```python
from build123d import *

# Parameters (mm, degrees)
SKETCH1_R           = 1.5
BOSS_EXTRUDE1_DEPTH = 3
BOSS_EXTRUDE2_START = 22.5
SKETCH2_W           = 3.5
SKETCH2_H           = 6
BOSS_EXTRUDE2_DEPTH = 29
SKETCH4_R           = 1.5
BOSS_EXTRUDE5_DEPTH = 1
CHAMFER2_SIZE       = 2
CHAMFER2_SIZE2      = 3.464101615
SKETCH3_W           = 24
SKETCH3_H           = 29
SKETCH3_R           = 11
BOSS_EXTRUDE4_DEPTH = 7
CHAMFER3_SIZE       = 2
SKETCH5_R           = 2
BOSS_EXTRUDE6_DEPTH = 14
CHAMFER5_SIZE       = 5


# Read off the part's stored shape, not the designer's step: Mirror1
with BuildPart() as part:
    # Sketch1 → Boss-Extrude1 (new body)
    with BuildSketch(Plane(origin=(0, 0, 0), x_dir=(1, 0, 0), z_dir=(0, 1, 0))):
        Polygon((-6, 17), (-3, 20), (3, 20), (6, 17), (6, -17), (3, -20), (-3, -20), (-6, -17), align=None)
        with Locations(Location((0, 14, 0), (0, 0, 270))):
            Circle(SKETCH1_R, mode=Mode.SUBTRACT)
        with Locations(Location((0, -14, 0), (0, 0, 270))):
            Circle(SKETCH1_R, mode=Mode.SUBTRACT)
    extrude(amount=BOSS_EXTRUDE1_DEPTH)

    # Sketch2 → Boss-Extrude2 (add)
    with BuildSketch(Plane(origin=(0, 3, 0), x_dir=(1, 0, 0), z_dir=(0, 1, 0)).offset(BOSS_EXTRUDE2_START)):
        with Locations((-7.75, 9)):
            Rectangle(SKETCH2_W, SKETCH2_H)
        with Locations((-7.75, -9)):
            Rectangle(SKETCH2_W, SKETCH2_H)
    extrude(amount=-BOSS_EXTRUDE2_DEPTH)

    # Sketch4 → Boss-Extrude5 (add)
    with BuildSketch(Plane(origin=(0, 3, 0), x_dir=(1, 0, 0), z_dir=(0, 1, 0))):
        Polygon((-3, 20), (-6, 17), (-6, 12), (-6, 6), (-6, -6), (-6, -12), (-6, -17), (-3, -20), (3, -20), (6, -17), (6, 17), (3, 20), align=None)
        with Locations(Location((0, 14, 0), (0, 0, 270))):
            Circle(SKETCH4_R, mode=Mode.SUBTRACT)
        with Locations(Location((0, -14, 0), (0, 0, 270))):
            Circle(SKETCH4_R, mode=Mode.SUBTRACT)
    extrude(amount=BOSS_EXTRUDE5_DEPTH)

    # Chamfer2
    chamfer2_edges = [part.edges().sort_by_distance(p)[0] for p in [
        (-6, 0, -9),
        (-6, 0, 9),
    ]]
    chamfer2_side = [part.faces().sort_by_distance(p)[0] for p in [
        (0, 0, 0),
    ]]
    chamfer(chamfer2_edges, length=CHAMFER2_SIZE, length2=CHAMFER2_SIZE2, reference=chamfer2_side[0])

    # Sketch3 → Boss-Extrude4 (add)
    with BuildSketch(Plane.ZY.offset(9.5)):
        with Locations((0, 11)):
            Rectangle(SKETCH3_W, SKETCH3_H)
        with Locations(Location((0, 11, 0), (0, 0, 236.944268849))):
            Circle(SKETCH3_R, mode=Mode.SUBTRACT)
    extrude(amount=BOSS_EXTRUDE4_DEPTH)

    # Chamfer3
    chamfer3_edges = [part.edges().sort_by_distance(p)[0] for p in [
        (-11.25, 25.5, -12),
        (-11.25, -3.5, -12),
        (-11.25, -3.5, 12),
        (-11.25, 25.5, 12),
    ]]
    chamfer(chamfer3_edges, length=CHAMFER3_SIZE)

    # Mirror1: part across plane


with BuildPart() as part_1:
    add(part.part)
    add(part.part.mirror(Plane(origin=(0, 11, 0), x_dir=(0, 0, 1), z_dir=(0, -1, 0))))

    # Sketch5 → Boss-Extrude6 (add)
    # profile 1 of 2: a face of its own
    with BuildSketch(Plane(origin=(0, 4, 0), x_dir=(1, 0, 0), z_dir=(0, 1, 0))):
        Polygon((6, -6), (-6, -6), (-6, -17), (-3, -20), (3, -20), (6, -17), align=None)
        with Locations(Location((0, -14, 0), (0, 0, 90))):
            Circle(SKETCH5_R, mode=Mode.SUBTRACT)
    # profile 2 of 2: a face of its own
    with BuildSketch(Plane(origin=(0, 4, 0), x_dir=(1, 0, 0), z_dir=(0, 1, 0))):
        Polygon((-6, 17), (-6, 6), (6, 6), (6, 17), (3, 20), (-3, 20), align=None)
        with Locations(Location((0, 14, 0), (0, 0, 90))):
            Circle(SKETCH5_R, mode=Mode.SUBTRACT)
    extrude(amount=BOSS_EXTRUDE6_DEPTH)

    # Chamfer5
    chamfer5_edges = [part_1.edges().sort_by_distance(p)[0] for p in [
        (-6, 11, 12),
        (-6, 11, -12),
    ]]
    chamfer(chamfer5_edges, length=CHAMFER5_SIZE - 0.0001)  # a hair under: the kernel refuses the full size


solid = part_1.part
```
For this review, take the finished solid that the model builds, in its own axes (mm). A direction names the side the tool comes from. Give positions to 0.01 mm unless a question says otherwise; leave off trailing zeros. Write each loop counter-clockwise with the first axis right and the second up, starting at its lowest first coordinate (ties: lowest second). Pieces come first, ordered by that corner, then holes.
Item 1: Take a section at A-A (y = 11). Give the number of separate pieces and of enclosed holes in the cut face, and give its area (3 significant figures).
Item 2: Take a section at D-D (x = -6.5). Give the boundary of the cut face in (y, z).
Item 3: Machinability: for faces 1 (the face through (0, 18, 0)), 2 (the face through (-9.5, 23, 0)), 3 (the face through (1.2, 10.9, -12.4)), which of the approach directions +Z, -Z, +X, -X, +Y, -Y give a long, thin tool a straight path to every point of the face, cutting with its end or side? Answer none if there is none.
Item 4: The part is to be moulded in two halves that separate along Y. For faces 4 (the face through (4, 11, 19)), 5 (the face through (1.2, 10.9, 15.6)), 6 (the face through (0, 22, 0)), 7 (the face through (-12, -3.5, 0)), say which applies: +Y half, -Y half, draft (parallel to the pull), parting line (faces both ways), or undercut.
Item 5: Wall thickness on probe 1 along Y at (x, z) = (4.75, 2); probe 2 along Y at (x, z) = (-12.5, 0); probe 3 along Y at (x, z) = (2.5, -18): over which ranges is each line inside the solid? List them lowest first.
Item 6: Take a section at C-C (z = 4). Give the boundary of the cut face in (x, y).
Item 7: Insertion check: P1, Ø1, axis at x = -7, y = 3.5, coming from the +Z side; P2, Ø5, axis at x = -5.5, z = -13.5, coming from the -Y side; P3, Ø4, axis at y = 14, z = -7.5, coming from the -X side. Each pin has a flat end and moves straight along its axis. Give the tip position at first contact, or say it passes through.
Established:
1. separate pieces: 2
1. enclosed holes: 2
1. area: 374 mm2
2. outline: (-3.5, -10) - (-1.5, -12) - (0, -12) - (0, -16.5) - (22, -16.5) - (22, -12) - (23.5, -12) - (25.5, -10) - (25.5, -6) - (-3.5, -6) - close; (-3.5, 6) - (25.5, 6) - (25.5, 10) - (23.5, 12) - (22, 12) - (22, 16.5) - (0, 16.5) - (0, 12) - (-1.5, 12) - (-3.5, 10) - close
3. face 1: +X, -X
3. face 2: +Y, -Y
3. face 3: none
4. face 4: draft
4. face 5: undercut
4. face 6: +Y half
4. face 7: -Y half
5. probe 1: y = 0 to 4, 18 to 22
5. probe 2: y = -3.5 to 0, 22 to 25.5
5. probe 3: y = 0 to 22
6. outline: (-16.5, -3.5) - (-9.5, -3.5) - (-9.5, 0.75) - (-16.5, 0.75) - close; (-16.5, 21.25) - (-9.5, 21.25) - (-9.5, 25.5) - (-16.5, 25.5) - close; (-6, 0) - (6, 0) - (6, 4) - (-6, 4) - close; (-6, 18) - (6, 18) - (6, 22) - (-6, 22) - close
7. P1: stops at z = 16.5
7. P2: stops at y = -2.5
7. P3: stops at x = -9.5
